Autodesk Inventor part; units mm, degrees
ref_plane "YZ Plane" through (0, 0, 0) normal (1, 0, 0) x (0, 1, 0)
ref_plane "XZ Plane" through (0, 0, 0) normal (0, 1, 0) x (-1, 0, 0)
ref_plane "XY Plane" through (0, 0, 0) normal (0, 0, 1) x (1, 0, 0)
sketch "Sketch1" plane through (0, 0, 0) normal (0, 1, 0) x (-1, 0, 0)
  circle A0 centre (0, 0) radius 1.65
  line L0 (0, 0) -> (0, -16) construction
  line L1 (-7, 0) -> (-7, -16)
  line L2 (7, -16) -> (7, 0)
  arc A1 (7, 0) -> (-7, 0) centre (0, 0) ccw
  arc A2 (-7, -16) -> (7, -16) centre (0, -16) ccw
  circle A3 centre (0, -16) radius 2.15
  point P0 (0, -8)
  dimension "d0" = 3.3
  dimension "d1" = 16
  dimension "d2" = 14
  dimension "d3" = 4.3
extrude "Extrusion1" add sketch "Sketch1" along normal blind 7
sketch "Sketch2" plane through (0, 0, 0) normal (0, -1, 0) x (1, 0, 0)
  circle A0 centre (0, 0) radius 1.65
  circle A1 centre (0, 0) radius 2.9
  dimension "d6" = 5.8
extrude "Extrusion2" cut sketch "Sketch2" against normal blind 3.2
mirror "Mirror1" about plane through (0, 0, 0) normal (0, 0, 1) of "Extrusion1", "Extrusion2"
ref_plane "Work Plane1" through (0, 0, 0) normal (0, 0, 1) x (1, 0, 0)
properties part number "futek-holder"
Geometry: final body of the model. Coordinates: model frame, mm. A direction names the side the tool comes from. Round coordinates to 2 decimals unless told otherwise and drop trailing zeros. Loops run counter-clockwise (first coordinate to the right, second up) from the corner with the lowest first, then second, coordinate; pieces in that order, holes last. Notation, with made-up numbers: (1.5, -6) -> (44.5, -6) arc R16 cw to (44.5, 13) -> close; hole circle Ø11 at (-39, 81.5). An arc over 180 degrees is marked (long way). Use one line per item in the form item = value.
Item 1: Cut plane B-B on x = 0. Output: boundary loops of the cut face in (y, z), then the cut area to 3 significant figures.
Evaluation:
outline = (0, -23) -> (7, -23) -> (7, -18.15) -> (0, -18.15) -> close; (0, -13.85) -> (7, -13.85) -> (7, -1.65) -> (3.2, -1.65) -> (3.2, -2.9) -> (0, -2.9) -> close; (0, 2.9) -> (3.2, 2.9) -> (3.2, 1.65) -> (7, 1.65) -> (7, 13.85) -> (0, 13.85) -> close; (0, 18.15) -> (7, 18.15) -> (7, 23) -> (0, 23) -> close
area = 231 mm2
Item 2: Cut plane D-D on y = 1. Output: boundary loops of the cut face in (x, z).
Evaluation:
outline = (-7, -16) arc R7 ccw to (7, -16) -> (7, 16) arc R7 ccw to (-7, 16) -> close; hole circle Ø5.8 at (0, 0); hole circle Ø4.3 at (0, -16); hole circle Ø4.3 at (0, 16)
Item 3: Material intervals for probe 1 along Z at (x, y) = (0, 5); probe 2 along Z at (x, y) = (0, 1.45); probe 3 along X at (y, z) = (4.5, 16), sorted ascending.
Evaluation:
probe_1 = -23 to -18.15, -13.85 to -1.65, 1.65 to 13.85, 18.15 to 23
probe_2 = -23 to -18.15, -13.85 to -2.9, 2.9 to 13.85, 18.15 to 23
probe_3 = -7 to -2.15, 2.15 to 7
Item 4: Contact query for flat-ended pins moving along their axis: pin 1 Ø4 at (x, z) = (0, 16) entering from -Y; pin 2 Ø1.5 at (x, y) = (4.5, 3) entering from +Z. Output: stop coordinate, or through.
Evaluation:
pin_1 = through
pin_2 = 21.91
Item 5: Cut plane C-C on y = 4.5. Output: boundary loops of the cut face in (x, z).
Evaluation:
outline = (-7, -16) arc R7 ccw to (7, -16) -> (7, 16) arc R7 ccw to (-7, 16) -> close; hole circle Ø4.3 at (0, -16); hole circle Ø4.3 at (0, 16); hole circle Ø3.3 at (0, 0)
Item 6: Access query for faces 1 (the flat face through (0, 3.2, 2)), 2 (the cylindrical face through (0.47, 3.45, 18.1)). Directions: +Z, -Z, +X, -X, +Y, -Y. A direction counts if a zero-diameter tool reaches every point of the face in a straight line with its end or side. Return the directions, or none.
Evaluation:
face_1 = -Y
face_2 = +Y, -Y
Item 7: Draft query along Z for faces 3 (the flat face through (3.2, 0, 0.3)), 4 (the cylindrical face through (0, 3, -23)), 5 (the cylindrical face through (0, 3, 23)), 6 (the cylindrical face through (-2.9, 1.6, 0.1)). Return one class per face: released by +Z, released by -Z, zero draft, split by the parting line, or undercut.
Evaluation:
face_3 = zero draft
face_4 = released by -Z
face_5 = released by +Z
face_6 = undercut
Item 8: Cut plane A-A on z = 0. Output: boundary loops of the cut face in (x, y).
Evaluation:
outline = (-7, 0) -> (-2.9, 0) -> (-2.9, 3.2) -> (-1.65, 3.2) -> (-1.65, 7) -> (-7, 7) -> close; (1.65, 3.2) -> (2.9, 3.2) -> (2.9, 0) -> (7, 0) -> (7, 7) -> (1.65, 7) -> close
